from build123d import *

# Parameters (mm, degrees)
SKETCH1_R           = 76
SKETCH1_W           = 100
SKETCH1_H           = 100
BOSS_EXTRUDE1_DEPTH = 5
SKETCH2_R           = 2.25
CUT_EXTRUDE1_DEPTH  = 10
SKETCH5_R           = 73
SKETCH5_R_2         = 70.710678119
BOSS_EXTRUDE3_DEPTH = 5
BOSS_EXTRUDE6_DEPTH = 10
CUT_EXTRUDE4_DEPTH  = 30
CUT_EXTRUDE5_DEPTH  = 70
BOSS_EXTRUDE7_DEPTH = 5
SKETCH14_R          = 1.5
CUT_EXTRUDE6_DEPTH  = 44
CUT_EXTRUDE7_DEPTH  = 30
SKETCH17_R          = 2.25
BOSS_EXTRUDE9_DEPTH = 5


with BuildPart() as part:
    # Sketch1 → Boss-Extrude1 (new body)
    with BuildSketch(Plane(origin=(0, 0, 0), x_dir=(1, 0, 0), z_dir=(0, 1, 0))):
        with Locations(Location((0, 0, 0), (0, 0, 270))):
            Circle(SKETCH1_R)
        Rectangle(SKETCH1_W, SKETCH1_H, mode=Mode.SUBTRACT)
    extrude(amount=BOSS_EXTRUDE1_DEPTH)

    # Sketch2 → Cut-Extrude1 (cut)
    with BuildSketch(Plane(origin=(0, 5, 0), x_dir=(1, 0, 0), z_dir=(0, 1, 0))):
        with Locations(Location((-62.5, 0, 0), (0, 0, 270))):
            Circle(SKETCH2_R)
        with Locations(Location((0, 62.5, 0), (0, 0, 270))):
            Circle(SKETCH2_R)
        with Locations(Location((62.5, 0, 0), (0, 0, 270))):
            Circle(SKETCH2_R)
        with Locations(Location((0, -62.5, 0), (0, 0, 270))):
            Circle(SKETCH2_R)
    extrude(amount=-CUT_EXTRUDE1_DEPTH, mode=Mode.SUBTRACT)

    # Sketch5 → Boss-Extrude3 (add)
    with BuildSketch(Plane(origin=(0, 5, 0), x_dir=(1, 0, 0), z_dir=(0, 1, 0))):
        with Locations(Location((0, 0, 0), (0, 0, 270))):
            Circle(SKETCH5_R)
        with Locations(Location((0, 0, 0), (0, 0, 135))):
            Circle(SKETCH5_R_2, mode=Mode.SUBTRACT)
    extrude(amount=BOSS_EXTRUDE3_DEPTH)

    # Sketch10 → Boss-Extrude6 (add)
    with BuildSketch(Plane(origin=(0, 5, 0), x_dir=(1, 0, 0), z_dir=(0, 1, 0))):
        with BuildLine():
            Line((3.25, -62.5), (3.25, -72.927618225))
            ThreePointArc((3.25, -72.927618225), (8.269673379, -72.530079982), (13.25, -71.787446674))
            Line((13.25, -71.787446674), (13.25, -62.5))
            Line((13.25, -62.5), (3.25, -62.5))
        make_face()
        with BuildLine():
            Line((-13.25, 62.5), (-3.25, 62.5))
            Line((-3.25, 62.5), (-3.25, 70.635950478))
            ThreePointArc((-3.25, 70.635950478), (-8.270990945, 70.225285395), (-13.25, 69.458170866))
            Line((-13.25, 69.458170866), (-13.25, 62.5))
        make_face()
        with BuildLine():
            ThreePointArc((-13.25, 69.458170866), (-8.270990945, 70.225285395), (-3.25, 70.635950478))
            Line((-3.25, 70.635950478), (-3.25, 72.927618225))
            ThreePointArc((-3.25, 72.927618225), (-8.269673379, 72.530079982), (-13.25, 71.787446674))
            Line((-13.25, 71.787446674), (-13.25, 69.458170866))
        make_face()
    extrude(amount=BOSS_EXTRUDE6_DEPTH)

    # Sketch11 → Cut-Extrude4 (cut)
    with BuildSketch(Plane.XY.offset(-62.5)):
        with BuildLine():
            ThreePointArc((-6.75, 10), (-7.189339828, 11.060660172), (-8.25, 11.5))
            Line((-8.25, 11.5), (-8.25, 8.5))
            ThreePointArc((-8.25, 8.5), (-7.189339828, 8.939339828), (-6.75, 10))
        make_face()
        with BuildLine():
            Line((-8.25, 8.5), (-8.25, 11.5))
            ThreePointArc((-8.25, 11.5), (-9.75, 10), (-8.25, 8.5))
        make_face()
    extrude(amount=-CUT_EXTRUDE4_DEPTH, mode=Mode.SUBTRACT)

    # Sketch12 → Cut-Extrude5 (cut)
    with BuildSketch(Plane(origin=(0, 0, 62.5), x_dir=(-1, 0, 0), z_dir=(0, 0, -1))):
        with BuildLine():
            ThreePointArc((-6.75, 10), (-7.189339828, 11.060660172), (-8.25, 11.5))
            Line((-8.25, 11.5), (-8.25, 8.5))
            ThreePointArc((-8.25, 8.5), (-7.189339828, 8.939339828), (-6.75, 10))
        make_face()
        with BuildLine():
            Line((-8.25, 8.5), (-8.25, 11.5))
            ThreePointArc((-8.25, 11.5), (-9.75, 10), (-8.25, 8.5))
        make_face()
    extrude(amount=-CUT_EXTRUDE5_DEPTH, mode=Mode.SUBTRACT)

    # Sketch13 → Boss-Extrude7 (add)
    with BuildSketch(Plane(origin=(0, 5, 0), x_dir=(1, 0, 0), z_dir=(0, 1, 0))):
        with BuildLine():
            Line((-62.5, -13.25), (-62.5, -3.25))
            Line((-62.5, -3.25), (-72.927618225, -3.25))
            ThreePointArc((-72.927618225, -3.25), (-72.530079982, -8.269673379), (-71.787446674, -13.25))
            Line((-71.787446674, -13.25), (-62.5, -13.25))
        make_face()
        with BuildLine():
            Line((-72.927618225, 3.25), (-62.5, 3.25))
            Line((-62.5, 3.25), (-62.5, 13.25))
            Line((-62.5, 13.25), (-71.787446674, 13.25))
            ThreePointArc((-71.787446674, 13.25), (-72.530079982, 8.269673379), (-72.927618225, 3.25))
        make_face()
        with BuildLine():
            Line((71.787446674, 13.25), (62.5, 13.25))
            Line((62.5, 13.25), (62.5, 3.25))
            Line((62.5, 3.25), (72.927618225, 3.25))
            ThreePointArc((72.927618225, 3.25), (72.530079982, 8.269673379), (71.787446674, 13.25))
        make_face()
        with BuildLine():
            Line((62.5, -3.25), (62.5, -13.25))
            Line((62.5, -13.25), (71.787446674, -13.25))
            ThreePointArc((71.787446674, -13.25), (72.530079982, -8.269673379), (72.927618225, -3.25))
            Line((72.927618225, -3.25), (62.5, -3.25))
        make_face()
    extrude(amount=BOSS_EXTRUDE7_DEPTH)

    # Sketch14 → Cut-Extrude6 (cut)
    with BuildSketch(Plane(origin=(0, 10, 0), x_dir=(1, 0, 0), z_dir=(0, 1, 0))):
        with BuildLine():
            ThreePointArc((-64.479085433, 8.25), (-64.918425261, 9.310660172), (-65.979085433, 9.75))
            Line((-65.979085433, 9.75), (-65.979085433, 6.75))
            ThreePointArc((-65.979085433, 6.75), (-64.918425261, 7.189339828), (-64.479085433, 8.25))
        make_face()
        with BuildLine():
            Line((-65.979085433, 6.75), (-65.979085433, 9.75))
            ThreePointArc((-65.979085433, 9.75), (-67.479085433, 8.25), (-65.979085433, 6.75))
        make_face()
        with BuildLine():
            ThreePointArc((-65.979085433, -6.75), (-67.479085433, -8.25), (-65.979085433, -9.75))
            Line((-65.979085433, -9.75), (-65.979085433, -6.75))
        make_face()
        with BuildLine():
            Line((-65.979085433, -6.75), (-65.979085433, -9.75))
            ThreePointArc((-65.979085433, -9.75), (-64.918425261, -9.310660172), (-64.479085433, -8.25))
            ThreePointArc((-64.479085433, -8.25), (-64.918425261, -7.189339828), (-65.979085433, -6.75))
        make_face()
        with Locations(Location((65.979085433, 8.25, 0), (0, 0, 270))):
            Circle(SKETCH14_R)
        with Locations(Location((65.979085433, -8.25, 0), (0, 0, 270))):
            Circle(SKETCH14_R)
    extrude(amount=-CUT_EXTRUDE6_DEPTH, mode=Mode.SUBTRACT)

    # Sketch16 → Cut-Extrude7 (cut)
    with BuildSketch(Plane(origin=(0, 5, 0), x_dir=(1, 0, 0), z_dir=(0, 1, 0))):
        with BuildLine():
            ThreePointArc((-30, -50), (-20, -60), (-10, -50))
            Line((-10, -50), (-30, -50))
        make_face()
        with BuildLine():
            Line((30, -50), (10, -50))
            ThreePointArc((10, -50), (20, -60), (30, -50))
        make_face()
        with BuildLine():
            Line((-30, 50), (-10, 50))
            ThreePointArc((-10, 50), (-20, 60), (-30, 50))
        make_face()
        with BuildLine():
            ThreePointArc((10, 50), (20, 60), (30, 50))
            Line((30, 50), (10, 50))
        make_face()
    extrude(amount=-CUT_EXTRUDE7_DEPTH, mode=Mode.SUBTRACT)

    # Sketch17 → Boss-Extrude9 (add)
    # profile 1 of 2: a face of its own
    with BuildSketch(Plane(origin=(0, 5, 0), x_dir=(1, 0, 0), z_dir=(0, 1, 0))):
        with BuildLine():
            Line((-62.5, -3.25), (-62.5, -13.25))
            ThreePointArc((-62.5, -13.25), (-54.514590429, 0), (-62.5, 13.25))
            Line((-62.5, 13.25), (-62.5, 3.25))
            Line((-62.5, 3.25), (-70.635950478, 3.25))
            ThreePointArc((-70.635950478, 3.25), (-70.710678119, 0), (-70.635950478, -3.25))
            Line((-70.635950478, -3.25), (-62.5, -3.25))
        make_face()
        with Locations(Location((-62.5, 0, 0), (0, 0, 270))):
            Circle(SKETCH17_R, mode=Mode.SUBTRACT)
    # profile 2 of 2: a face of its own
    with BuildSketch(Plane(origin=(0, 5, 0), x_dir=(1, 0, 0), z_dir=(0, 1, 0))):
        with BuildLine():
            Line((62.5, -3.25), (62.5, -13.25))
            ThreePointArc((62.5, -13.25), (54.514590429, 0), (62.5, 13.25))
            Line((62.5, 13.25), (62.5, 3.25))
            Line((62.5, 3.25), (70.635950478, 3.25))
            ThreePointArc((70.635950478, 3.25), (70.710678119, 0), (70.635950478, -3.25))
            Line((70.635950478, -3.25), (62.5, -3.25))
        make_face()
        with Locations(Location((62.5, 0, 0), (0, 0, 270))):
            Circle(SKETCH17_R, mode=Mode.SUBTRACT)
    extrude(amount=BOSS_EXTRUDE9_DEPTH)


solid = part.part
Build history of the part. All positions in model axes, mm. A direction names the side the tool comes from. Round coordinates to 2 decimals unless told otherwise and drop trailing zeros. Write each loop counter-clockwise with the first axis right and the second up, starting at its lowest first coordinate (ties: lowest second). Pieces come first, ordered by that corner, then holes. Notation, with made-up numbers: M 18,-31 L 68,-31 A14 ccw 68,-14 Z; hole C 30,-5 d11. An arc over 180 degrees is marked long. Answer as a JSON object with one key per item and string values. Group by question number.
(1) Flat gauge pins, fed straight in: pin 1 (6 mm diameter, centred on x = 58.5, z = -19.5, fed in from +Y); pin 2 (8 mm diameter, centred on x = 6.5, z = -42.5, fed in from +Y); pin 3 (1.5 mm diameter, centred on y = 3, z = -11.5, fed in from -X); pin 4 (4 mm diameter, centred on x = 37.5, y = 3, fed in from -Z). Where does each tip first touch, or does it go through?
(2) Mould opens along X. For faces 3 (the cylindrical face through (-46.245, 2.465, -60.311)), 4 (the flat face through (1, 5, -58)), 5 (the flat face through (8, 15, 68)) say: pulls with the +X half, pulls with the -X half, needs draft (parallel to the pull), parting line crosses it, or undercut.
(3) Cut at A-A (z = -32). Give the cut face in (x, y), and give its area (3 significant figures).
(4) Which spindle directions (+Z, -Z, +X, -X, +Y, -Y) get a long thin tool onto all of the face, cutting with end or side? Do faces 1 (the flat face through (-40, 2, -50)), 2 (the flat face through (66, 7, 13.25)). Say none if no direction does.
(5) Drill centre lines: L1, parallel to X at y = 7.6, z = 0; L2, parallel to X at y = 3.75, z = -50.5; L3, parallel to X at y = 6.25, z = -8.25. Where is each one in solid material? Low to high.
(6) Cut at B-B (x = -28). Give the cut face in (y, z), and give its area (3 significant figures).
Responses:
{
 "1": {"pin 1": "stops at y = 5", "pin 2": "passes through", "pin 3": "stops at x = -75.24", "pin 4": "stops at z = -67.2"},
 "2": {"face 3": "parting line crosses it", "face 4": "undercut", "face 5": "needs draft"},
 "3": {"outline": "M -68.93,0 L -50,0 L -50,5 L -63.06,5 L -63.06,10 L -65.61,10 L -65.61,5 L -68.93,5 Z; M 50,0 L 68.93,0 L 68.93,5 L 65.61,5 L 65.61,10 L 63.06,10 L 63.06,5 L 50,5 Z", "area": "215 mm2"},
 "4": {"face 1": "+Y, -Y", "face 2": "+Y"},
 "5": {"L1": "x = -73 to -64.75, -60.25 to -54.51, 54.51 to 60.25, 64.75 to 73", "L2": "x = -56.8 to -29.99, -10.01 to 10.01, 29.99 to 56.8", "L3": "x = -72.53 to -67.48, -64.48 to -56.99, 56.99 to 64.48, 67.48 to 72.53"},
 "6": {"outline": "M 0,-70.65 L 5,-70.65 L 5,-67.42 L 10,-67.42 L 10,-64.93 L 5,-64.93 L 5,-56 L 0,-56 Z; M 0,56 L 5,56 L 5,64.93 L 10,64.93 L 10,67.42 L 5,67.42 L 5,70.65 L 0,70.65 Z", "area": "171 mm2"}
}
